Build history of the part. All positions in model axes, mm. Give positions to 0.01 mm unless a question says otherwise; leave off trailing zeros. Order: outer loops, then holes, each group sorted by start corner. A loop starts at its lowest first (then second) coordinate and runs counter-clockwise, first axis right, second up. Notation, with made-up numbers: (84, -3.5) -> (114, -3.5) arc R26 ccw to (114, 25.5) -> close; hole circle Ø10 at (-14.5, -13.75). An arc over 180 degrees is marked (long way). One line per item, written item: value. Start each with the question number.
(1) Saw through at A-A on y = 0. Give the cut face in (x, z), plus the area to 3 significant figures.
(2) Pin check, flat tips, straight feed: pin 1 (4 mm diameter, centred on x = -8.5, z = 18.5, fed in from -Y); pin 2 (5 mm diameter, centred on x = -9, z = 4.5, fed in from -Y); pin 3 (1.5 mm diameter, centred on x = 4, z = 5, fed in from +Y); pin 4 (10 mm diameter, centred on x = -10, y = 5.5, fed in from +Z). Stop position of each tip, or through.
(3) Two-plate mould, pull along X, no slides. Class faces 1 (the cylindrical face through (-10.11, -7.35, 18.41)), 2 (the flat face through (10.33, 5.57, 19.35)), 3 (the flat face through (2.786, -11.421, 19.351)), 4 (the cylindrical face through (2.17, -9.76, 8.96)): +X half, -X half, draft (parallel to the pull), parting line (faces both ways), or undercut.
(4) Saw through at C-C on z = 3.75. Give the cut face in (x, y), plus the area to 3 significant figures.
(5) Saw through at B-B on z = 7.25. Give the cut face in (x, y).
(6) Probe line 1 (X direction, y = 9.25, z = 14.75); line 2 (Y direction, x = -8.5, z = 17); line 3 (Z direction, x = 8, y = 7.25). List the from-to ranges inside material, lowest first.
```python
from build123d import *

# Parameters (mm, degrees)
F5_DEPTH        = 15
F5_COPIES_COUNT = 30


# Not quite as in the source:
# - a feature of the source that left no trace in its solid (it failed there, or was rolled back) is left out
# - a pattern or mirror of a feature is missing from the dataset's text; its kind, count and spacing are read off the source's solid


with BuildPart() as f3:
    # F2 (on Front) → F3 (revolve)
    with BuildSketch(Plane.XZ):
        with BuildLine():
            Line((-11.25, 0), (0, 0))
            Line((0, 0), (0, 27))
            Line((0, 27), (-10.5, 27))
            Line((-10.5, 27), (-12.5, 25))
            Line((-12.5, 25), (-12.5, 12))
            Line((-12.5, 12), (-10, 12))
            Line((-10, 12), (-10, 6))
            Line((-10, 6), (-11.25, 6))
            Line((-11.25, 6), (-11.25, 4.5))
            ThreePointArc((-11.25, 4.5), (-10.5728756555, 3), (-11.25, 1.5))
            Line((-11.25, 1.5), (-11.25, 0))
        make_face()
    revolve(axis=Axis((0, 0, 13.5), (0, 0, -1)))

    # F4 (on face) → F5 (cut)
    with BuildSketch(Plane.XY.offset(27)):
        with BuildLine():
            Line((0, 11), (0.6905599091, 12.4809105041))
            ThreePointArc((0.6905599091, 12.4809105041), (0, 12.5), (-0.6905599091, 12.4809105041))
            Line((-0.6905599091, 12.4809105041), (0, 11))
        make_face()
    f5 = extrude(amount=-F5_DEPTH, mode=Mode.SUBTRACT)

    # F5_copies: F5 ×30 about axis
    f5_copies_axis = Axis((0, 0, 0), (0, 0, 1))
    for i in range(1, F5_COPIES_COUNT):
        add(f5.rotate(f5_copies_axis, i * 360 / F5_COPIES_COUNT), mode=Mode.SUBTRACT)


solid = f3.part
```
Results below:
1. outline: (-12.5, 12) -> (-10, 12) -> (-10, 6) -> (-11.25, 6) -> (-11.25, 4.5) arc R2 cw to (-11.25, 1.5) -> (-11.25, 0) -> (11.25, 0) -> (11.25, 1.5) arc R2 cw to (11.25, 4.5) -> (11.25, 6) -> (10, 6) -> (10, 12) -> (12.5, 12) -> (12.5, 25) -> (10.5, 27) -> (-10.5, 27) -> (-12.5, 25) -> close
1. area: 623 mm²
2. pin 1: stops at y = -10.68
2. pin 2: stops at y = -9.18
2. pin 3: stops at y = 10.77
2. pin 4: stops at z = 27
3. face 1: -X half
3. face 2: undercut
3. face 3: undercut
3. face 4: parting line
4. outline: circle Ø21.44 at (0, 0)
4. area: 361 mm²
5. outline: circle Ø20 at (0, 0)
6. line 1: x = -8.41 to -7.1, -6.53 to 6.53, 7.1 to 8.41
6. line 2: y = -9.17 to -8.13, -7.46 to 7.46, 8.13 to 9.17
6. line 3: z = 0 to 2.08, 3.92 to 6, 12 to 26.7
